from build123d import *

# Parameters (mm, degrees)
F0_W      = 27
F0_H      = 12
F1_DEPTH  = 12.5
F3_DEPTH  = 3.25
F5_DEPTH  = 3.5
F6_R      = 6
F7_DEPTH  = 25
F8_R      = 1.75
F9_DEPTH  = 25
F10_W     = 12
F10_H     = 0.5
F11_DEPTH = 31
F12_R     = 1


with BuildPart() as f1:
    # F0 (on Top) → F1 (new body)
    with BuildSketch(Plane.XY):
        Rectangle(F0_W, F0_H)
    extrude(amount=-F1_DEPTH)

    # F2 (on face) → F3 (cut)
    with BuildSketch(Plane.XZ.offset(6)):
        with BuildLine():
            Line((8, 0), (-8, 0))
            ThreePointArc((-8, 0), (0, -8), (8, 0))
        make_face()
    extrude(amount=-F3_DEPTH, mode=Mode.SUBTRACT)

    # F4 (on face) → F5 (cut)
    with BuildSketch(Plane(origin=(0, 6, 0), x_dir=(-1, 0, 0), z_dir=(0, 1, 0))):
        with BuildLine():
            Line((8, 0), (-8, 0))
            ThreePointArc((-8, 0), (0, -8), (8, 0))
        make_face()
    extrude(amount=-F5_DEPTH, mode=Mode.SUBTRACT)

    # F6 (on face) → F7 (cut)
    with BuildSketch(Plane(origin=(0, 2.5, 0), x_dir=(-1, 0, 0), z_dir=(0, 1, 0))):
        Circle(F6_R)
    extrude(amount=-F7_DEPTH, mode=Mode.SUBTRACT)

    # F8 (on face) → F9 (cut)
    with BuildSketch(Plane.XY):
        with Locations((10.5, 0)):
            Circle(F8_R)
        with Locations((-10.5, 0)):
            Circle(F8_R)
    extrude(amount=-F9_DEPTH, mode=Mode.SUBTRACT)

    # F10 (on face) → F11 (cut)
    with BuildSketch(Plane(origin=(-13.5, 0, 0), x_dir=(0, -1, 0), z_dir=(-1, 0, 0))):
        with Locations((0, -0.25)):
            Rectangle(F10_W, F10_H)
    extrude(amount=-F11_DEPTH, mode=Mode.SUBTRACT)

    # F12
    f12_edges = [f1.edges().sort_by_distance(p)[0] for p in [
        (-13.5, -6, -6.5),
        (-13.5, 6, -6.5),
        (-13.5, 0, -12.5),
        (0, -6, -12.5),
        (0, 6, -12.5),
        (13.5, -6, -6.5),
        (13.5, 6, -6.5),
        (13.5, 0, -12.5),
    ]]
    fillet(f12_edges, radius=F12_R)


solid = f1.part
Work out the finished part from the listing and answer in its coordinate system (mm). A direction names the side the tool comes from. Give positions to 0.01 mm unless a question says otherwise; leave off trailing zeros. Loops run counter-clockwise (first coordinate to the right, second up) from the corner with the lowest first, then second, coordinate; pieces in that order, holes last. Notation, with made-up numbers: (81.25, 42) -> (102.25, 42) arc R23 ccw to (102.25, 50) -> close; hole circle Ø7 at (78.25, 54.25). An arc over 180 degrees is marked (long way). Use a Markdown table: item, result. Add a question column.
1. Section D-D on x = 0 is taken. Determine the outline of the cut face in (y, z), and give its area (3 significant figures).
2. For faces 1 (the cylindrical face through (0, -4, -8)), 2 (the cylindrical face through (0, 4, -8)), 3 (the cylindrical face through (0, 0, -6)), determine the directions among +Z, -Z, +X, -X, +Y, -Y from which every point of the face is accessible in a straight line to the end or side of a thin tool.
3. Section A-A on x = -10.5 is taken. Determine the outline of the cut face in (y, z), and give its area (3 significant figures).
4. Section C-C on z = -9.25 is taken. Determine the outline of the cut face in (x, y).
5. Determine the mould class of faces 4 (the cylindrical face through (-13.215, -5.699, -6.077)), 5 (the cylindrical face through (13.199, 5.715, -6.077)), 6 (the cylindrical face through (-8.831, 0.526, -6.416)), 7 (the flat face through (-0.2, 6, -8.4)) for opening direction X: released by +X, released by -X, zero draft, split by the parting line, or undercut.
6. Find the intervals of material crossed by probe 1 along Y at (x, z) = (-10.5, -7.75); probe 2 along Y at (x, z) = (-9, -12); probe 3 along X at (y, z) = (-2, -3.5), in increasing order.
7. A flat-ended cylindrical pin translates along its axis: pin 1 Ø2 at (x, y) = (10.5, 0) entering from +Z. Find the tip coordinate at first contact, or state that the pin passes through.
8. Section B-B on y = 0 is taken. Determine the outline of the cut face in (x, z).
Results below:
| question | item | result |
|---|---|---|
| 1 | outline | (-6, -11.5) arc R1 ccw to (-5, -12.5) -> (5, -12.5) arc R1 ccw to (6, -11.5) -> (6, -8) -> (2.5, -8) -> (2.5, -6) -> (-2.75, -6) -> (-2.75, -8) -> (-6, -8) -> close |
| 1 | area | 64.1 mm^2 |
| 2 | face 1 | +Z, -Y |
| 2 | face 2 | +Z, +Y |
| 2 | face 3 | +Z, +Y, -Y |
| 3 | outline | (-6, -11.5) arc R1 ccw to (-5, -12.5) -> (-1.75, -12.5) -> (-1.75, -0.5) -> (-6, -0.5) -> close; (1.75, -12.5) -> (5, -12.5) arc R1 ccw to (6, -11.5) -> (6, -0.5) -> (1.75, -0.5) -> close |
| 3 | area | 102 mm^2 |
| 4 | outline | (-13.5, -5) arc R1 ccw to (-12.5, -6) -> (12.5, -6) arc R1 ccw to (13.5, -5) -> (13.5, 5) arc R1 ccw to (12.5, 6) -> (-12.5, 6) arc R1 ccw to (-13.5, 5) -> close; hole circle Ø3.5 at (-10.5, 0); hole circle Ø3.5 at (10.5, 0) |
| 5 | face 4 | released by -X |
| 5 | face 5 | released by +X |
| 5 | face 6 | undercut |
| 5 | face 7 | zero draft |
| 6 | probe 1 | y = -6 to -1.75, 1.75 to 6 |
| 6 | probe 2 | y = -5.87 to -0.9, 0.9 to 5.87 |
| 6 | probe 3 | x = -13.5 to -4.87, 4.87 to 13.5 |
| 7 | pin 1 | passes through |
| 8 | outline | (-13.5, -11.5) arc R1 ccw to (-12.5, -12.5) -> (-12.25, -12.5) -> (-12.25, -0.5) -> (-13.5, -0.5) -> close; (-8.75, -12.5) -> (8.75, -12.5) -> (8.75, -0.5) -> (5.98, -0.5) arc R6 cw to (-5.98, -0.5) -> (-8.75, -0.5) -> close; (12.25, -12.5) -> (12.5, -12.5) arc R1 ccw to (13.5, -11.5) -> (13.5, -0.5) -> (12.25, -0.5) -> close |
